from build123d import *

# Parameters (mm, degrees)
SKETCH1_R           = 7.14375
SKETCH1_R_2         = 2.413
BOSS_EXTRUDE1_DEPTH = 12.7
SKETCH2_R           = 4.05
CUT_EXTRUDE1_DEPTH  = 3
CUT_EXTRUDE2_START  = -3
SKETCH3_R           = 4.05
CUT_EXTRUDE2_DEPTH  = 3
FILLET1_R           = 0.79375


with BuildPart() as part:
    # Sketch1 → Boss-Extrude1 (new body)
    with BuildSketch(Plane.XY):
        Circle(SKETCH1_R)
        Circle(SKETCH1_R_2, mode=Mode.SUBTRACT)
    extrude(amount=BOSS_EXTRUDE1_DEPTH)

    # Sketch2 → Cut-Extrude1 (cut)
    with BuildSketch(Plane.XY.offset(12.7)):
        Circle(SKETCH2_R)
    extrude(amount=-CUT_EXTRUDE1_DEPTH, mode=Mode.SUBTRACT)

    # Sketch3 → Cut-Extrude2 (cut)
    with BuildSketch(Plane(origin=(0, 0, 0), x_dir=(-1, 0, 0), z_dir=(0, 0, -1)).offset(CUT_EXTRUDE2_START)):
        with Locations(Location((0, 0, 0), (0, 0, 180))):
            Circle(SKETCH3_R)
    extrude(amount=CUT_EXTRUDE2_DEPTH, mode=Mode.SUBTRACT)

    # Fillet1
    fillet1_edges = [part.edges().sort_by_distance(p)[0] for p in [
        (-7.14375, 0, 0),
        (-7.14375, 0, 12.7),
    ]]
    fillet(fillet1_edges, radius=FILLET1_R)


solid = part.part
For this review, take the finished solid that the model builds, in its own axes (mm). A direction names the side the tool comes from. Round coordinates to 2 decimals unless told otherwise and drop trailing zeros. Order: outer loops, then holes, each group sorted by start corner. A loop starts at its lowest first (then second) coordinate and runs counter-clockwise, first axis right, second up. Notation, with made-up numbers: M 82,22 L 111,22 A13 cw 111,28 Z; hole C 27.25,46 d6. An arc over 180 degrees is marked long. Use a Markdown table: item, result. Add a question column.
Item 1: Insertion check: pin 1 (1 mm diameter, centred on y = -2, z = 2, fed in from -X); pin 2 (3 mm diameter, centred on x = -2.5, z = 6.5, fed in from +Y); pin 3 (2.5 mm diameter, centred on x = 0.5, y = 0, fed in from +Z). Each pin has a flat end and moves straight along its axis. Give the tip position at first contact, or say it passes through.
Item 2: Add section C-C, the plane z = 1.5. Give the boundary of the cut face in (x, y), then the cut area to 3 significant figures.
Item 3: Add section D-D, the plane z = 6.5. Give the boundary of the cut face in (x, y).
Item 4: Add section A-A, the plane y = 0. Give the boundary of the cut face in (x, z), then the cut area to 4 significant figures.
Item 5: Tool access review of faces 4 (the cylindrical face through (-0.878, -3.954, 11.221)), 5 (the flat face through (2, 2, 3)), 6 (the cylindrical face through (-1.915, -1.468, 6.303)): name each direction out of +Z, -Z, +X, -X, +Y, -Y from which nothing blocks a thin tool from reaching the whole face with its end or side.
Item 6: To check wall thickness, follow line 1 along Y through (x, z) = (0, 5); line 2 along Y through (x, z) = (0, 0.95); line 3 along Z through (x, y) = (-3.25, -1.25). State the ranges of each line that lie inside material, in increasing order.
Item 7: Mouldability with a two-part tool opening along X and no side actions: class faces 1 (the cylindrical face through (-0.878, 3.954, 1.521)), 2 (the cylindrical face through (-7.137, 0.314, 6.272)), 3 (the flat face through (1.3, -4.1, 0)) as released by +X, released by -X, zero draft, split by the parting line, or undercut.
Geometry results:
| question | item | result |
|---|---|---|
| 1 | pin 1 | stops at x = -6.98 |
| 1 | pin 2 | stops at y = 7.07 |
| 1 | pin 3 | passes through |
| 2 | outline | C 0,0 d14.29; hole C 0,0 d8.1 |
| 2 | area | 109 mm² |
| 3 | outline | C 0,0 d14.29; hole C 0,0 d4.83 |
| 4 | outline | M -7.14,0.79 A0.79 ccw -6.35,0 L -4.05,0 L -4.05,3 L -2.41,3 L -2.41,9.7 L -4.05,9.7 L -4.05,12.7 L -6.35,12.7 A0.79 ccw -7.14,11.91 Z; M 2.41,3 L 4.05,3 L 4.05,0 L 6.35,0 A0.79 ccw 7.14,0.79 L 7.14,11.91 A0.79 ccw 6.35,12.7 L 4.05,12.7 L 4.05,9.7 L 2.41,9.7 Z |
| 4 | area | 100.0 mm² |
| 5 | face 4 | +Z |
| 5 | face 5 | -Z |
| 5 | face 6 | +Z, -Z |
| 6 | line 1 | y = -7.14 to -2.41, 2.41 to 7.14 |
| 6 | line 2 | y = -7.14 to -4.05, 4.05 to 7.14 |
| 6 | line 3 | z = 3 to 9.7 |
| 7 | face 1 | undercut |
| 7 | face 2 | split by the parting line |
| 7 | face 3 | zero draft |
